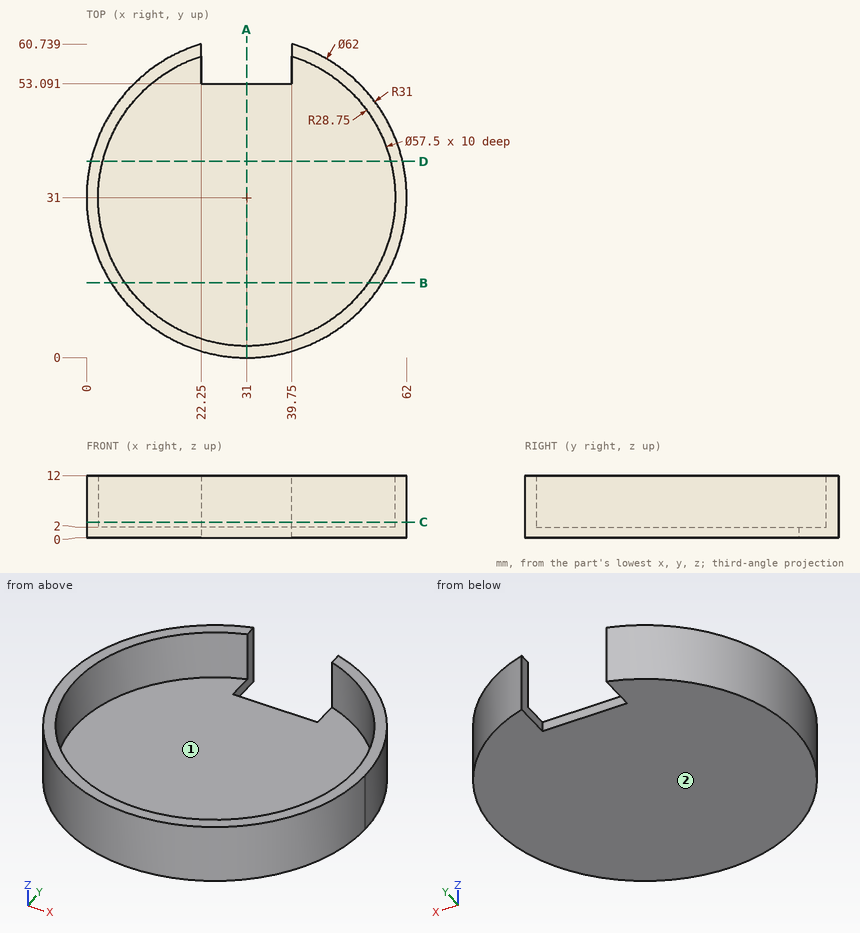
Study the drawing (mm; zero at the part's minimum x, y, z) and answer. A direction names the side the tool comes from. Coordinates: 2 decimals unless noted, no trailing zeros. Loops run counter-clockwise (first coordinate to the right, second up) from the corner with the lowest first, then second, coordinate; pieces in that order, holes last. Notation, with made-up numbers: (-15, 2.5) -> (11, 2.5) arc R26 ccw to (11, 37.5) -> close; hole circle Ø3 at (84.5, 38.5). An arc over 180 degrees is marked (long way). Answer in a Markdown table with one row per item. Add a question column.
1. The part is cut by section D-D, the plane y = 38. Write down the section's boundary in (x, z) (1 decimal), then the cut area to 3 significant figures.
2. Flat-ended cylindrical pins translate along their axes: P1, Ø3, axis at x = 15, z = 2.5, coming from the +Y side; P2, Ø3, axis at x = 11, z = 9, coming from the +Y side (1 decimal); P3, Ø1, axis at x = 34.5, z = 1.5, coming from the +Y side. Find the tip coordinate at first contact, or state that the pin passes through.
3. The part is cut by section C-C, the plane z = 3. Write down the section's boundary in (x, y).
4. For the marked faces 1 and 2, determine the directions among +Z, -Z, +X, -X, +Y, -Y from which every point of the face is accessible in a straight line to the end or side of a thin tool.
5. The part is cut by section A-A, the plane x = 31. Write down the section's boundary in (y, z), then the cut area to 3 significant figures.
6. The part is cut by section B-B, the plane y = 14.5. Write down the section's boundary in (x, z) (1 decimal).
7. Consider line 1 (Z direction, x = 37, y = 5.5); line 2 (X direction, y = 11, z = 3.25) (1 decimal); line 3 (Y direction, x = 55, z = 4.75) (1 decimal). Determine where each line is inside the solid, lowest interval first. Write a range as [from, to].
Answer below:
| question | item | result |
|---|---|---|
| 1 | outline | (0.8, 0) -> (61.2, 0) -> (61.2, 12) -> (58.9, 12) -> (58.9, 2) -> (3.1, 2) -> (3.1, 12) -> (0.8, 12) -> close |
| 1 | area | 167 mm2 |
| 2 | P1 | y = 58.4 |
| 2 | P2 | y = 55.9 |
| 2 | P3 | y = 53.09 |
| 3 | outline | (22.25, 58.39) -> (22.25, 60.74) arc R31 ccw (long way) to (39.75, 60.74) -> (39.75, 58.39) arc R28.75 cw (long way) to start |
| 4 | face 1 | +Z |
| 4 | face 2 | -Z, +X, -X, +Y, -Y |
| 5 | outline | (0, 0) -> (53.09, 0) -> (53.09, 2) -> (2.25, 2) -> (2.25, 12) -> (0, 12) -> close |
| 5 | area | 129 mm2 |
| 6 | outline | (4.8, 0) -> (57.2, 0) -> (57.2, 12) -> (54.5, 12) -> (54.5, 2) -> (7.5, 2) -> (7.5, 12) -> (4.8, 12) -> close |
| 7 | line 1 | [0, 2] |
| 7 | line 2 | [7.3, 10.3], [51.7, 54.7] |
| 7 | line 3 | [11.4, 15.2], [46.8, 50.6] |
